Autodesk Inventor part; units mm, degrees
ref_plane "YZ Plane" through (0, 0, 0) normal (1, 0, 0) x (0, 1, 0)
ref_plane "XZ Plane" through (0, 0, 0) normal (0, 1, 0) x (-1, 0, 0)
ref_plane "XY Plane" through (0, 0, 0) normal (0, 0, 1) x (1, 0, 0)
sketch "스케치1" plane through (0, 0, 0) normal (0, 1, 0) x (-1, 0, 0)
  line L0 (0, 0) -> (12, 0)
  line L1 (12, 0) -> (12, -4)
  line L2 (12, -4) -> (0, -4)
  line L3 (0, -4) -> (0, 0)
  dimension "d0" = 12
  dimension "d1" = 4
extrude "돌출1" add sketch "스케치1" along normal blind 3.5
sketch "스케치2" plane through (0, 3.5, 0) normal (0, 1, 0) x (1, 0, 0)
  line L0 (0, 0) -> (0, 4) construction
  line L1 (0, 2) -> (-12, 2) construction
  line L2 (-12, 4) -> (-12, 0) construction
  point P0 (-1.3, 2)
  point P1 (-7.7, 2)
  point P2 (-10.7, 2)
  dimension "d59" = 1.3
  dimension "d60" = 3
  dimension "d62" = 1.3
hole "구멍1" at (-10.7, 3.5, -2) at (-1.3, 3.5, -2) direction (0, -1, 0) diameter 1.1 end through all
hole "구멍2" at (-7.7, 3.5, -2) direction (0, -1, 0) diameter 1.1 end through all
sketch "스케치11" plane through (0, 0, -4) normal (0, 0, -1) x (-1, 0, 0)
  line L0 (0, 0) -> (12, 0)
  line L1 (0, 0) -> (0, 3.5)
  line L2 (12, 3.5) -> (0, 3.5)
  line L3 (12, 0) -> (12, 3.5)
  line L4 (12, 3.5) -> (0, 3.5)
  line L5 (2.5, 3.5) -> (4.1, 3.5)
  line L6 (4.1, 3.5) -> (4.1, -4)
  line L7 (4.1, -4) -> (2.5, -4)
  line L8 (2.5, -4) -> (2.5, 3.5)
  dimension "d99" = 1.6
  dimension "d100" = 4
  dimension "d124" = 2.5
extrude "돌출9" add sketch "스케치11" along normal blind 1.5 contours L8 L2 L6 L0 | L0 L6 L7 L8
chamfer "모따기6" distance 1 angle 45 2 edges at (-2.5, 1.75, -4) (-4.1, 1.75, -4)
chamfer "모따기7" distance 0.5 angle 45 2 edges at (-2.5, 0, -4.5) (-4.1, 0, -4.5)
sketch "스케치12" plane through (0, 0, -5.5) normal (0, 0, -1) x (-1, 0, 0)
  line L0 (4.1, 3.5) -> (2.5, 3.5)
  line L1 (2.5, 3.5) -> (2.5, -4)
  line L2 (2.5, -4) -> (4.1, -4)
  line L3 (4.1, -4) -> (4.1, 3.5)
  line L4 (2.8, -4) -> (2.8, 3.5)
  line L5 (12, 3.5) -> (0, 3.5)
  line L6 (3.8, 3.5) -> (3.8, -4)
  line L7 (2.5, -4) -> (4.1, -4)
  point P0 (0, 0)
  point P1 (3.8, -4)
  dimension "d110" = 1
  dimension "d111" = 0.3
  dimension "d112" = 0.3
extrude "돌출10" cut sketch "스케치12" against normal blind 0.2 contours L6 L2 L4 L0
sketch "스케치13" plane through (0, 0, -4) normal (0, 0, 1) x (1, 0, 0)
  line L0 (-4.6, 0) -> (-2, 0)
  line L1 (-4.1, -0.5) -> (-4.6, 0)
  line L2 (-4.1, -4) -> (-4.1, -0.5)
  line L3 (-2.5, -4) -> (-4.1, -4)
  line L4 (-2.5, -0.5) -> (-2.5, -4)
  line L5 (-2, 0) -> (-2.5, -0.5)
  point P0 (0, 0)
extrude "돌출11" cut sketch "스케치13" against normal blind 0.5
chamfer "모따기8" distance 0.5 distance2 1 1 edges at (-3.3, -4, -4.5) measured on face at (-3.1333, -4, -4.7667)
sketch "스케치14" plane through (-12, 0, 0) normal (0, 0, 1) x (1, 0, 0)
  line L0 (12, 0) -> (0, 0)
  line L1 (12, 0) -> (12, 3.5)
  line L2 (0, 3.5) -> (12, 3.5)
  line L3 (0, 0) -> (0, 3.5)
extrude "돌출12" cut sketch "스케치14" against normal blind 0.5
equation "\"d111\" = d112"
equation "\"G23_F\" = 0.65"
equation "\"G23_M\" = 0.67"
equation "\"Screw_F\" = 1.3"
equation "\"Screw_M\" = 1.6"
properties part number "_3D 인쇄"
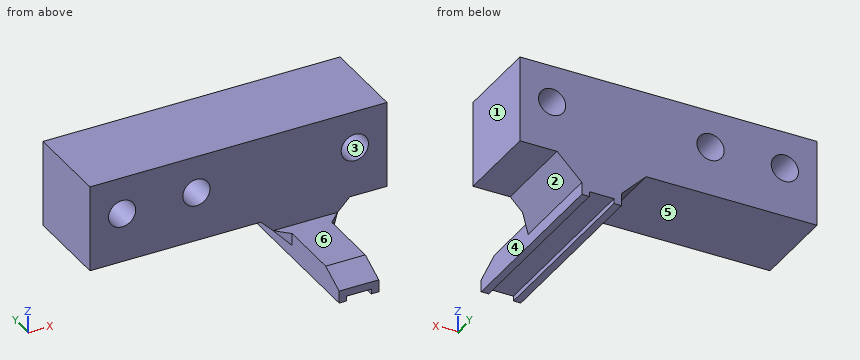
Verification items for the finished model (mm, model axes). Face numbers are marked on the shaded views. A direction names the side the tool comes from. Coordinates: 2 decimals unless noted, no trailing zeros. Order: outer loops, then holes, each group sorted by start corner. A loop starts at its lowest first (then second) coordinate and runs counter-clockwise, first axis right, second up. Notation, with made-up numbers: M 72.25,-35 L 130.25,-35 A37 cw 130.25,4 Z; hole C 60.25,-17 d2. An arc over 180 degrees is marked long. One line per item, written item: value. Start each with the question number.
Item 1: Sectioned sample at A-A (z = -2). Enter the section's corners in (x, y).
Item 2: Sectioned sample at C-C (y = -1). Enter the section's corners in (x, z).
Item 3: Scan lines: probe 1 along X at (y, z) = (2.65, -2); probe 2 along Z at (x, y) = (-10.7, 1.05); probe 3 along Z at (x, y) = (-7, 2). Record each from-to range of solid material in increasing order.
Item 4: Mould release check, pull along Z, two halves, no side actions. Record for the marked faces 1, 2 and 3: released by +Z, released by -Z, zero draft, split by the parting line, or undercut.
Item 5: Sectioned sample at B-B (x = -10.7). Enter the section's corners in (y, z), then the cut area to 3 significant figures.
Item 6: Gauge pin test, flat ends, axial feed: pin 1 (1.8 mm diameter, centred on x = -8, y = 2, fed in from -Z); pin 2 (3 mm diameter, centred on x = -3.5, y = -2, fed in from +Z); pin 3 (0.5 mm diameter, centred on y = -1.5, z = -5, fed in from -X). Record the tip position at first contact, or that the pin passes through.
Item 7: Access from +Z, -Z, +X, -X, +Y, -Y to the whole of each face (thin tool, end or side, straight path). Record for the marked faces 4, 5 and 6.
Item 8: Sectioned sample at D-D (y = 2.5). Enter the section's corners in (x, z), then the cut area to 3 significant figures.
Conclusion:
1. outline: M -12,0 L -11.25,0 L -11.25,3.5 L -12,3.5 Z; M -10.15,0 L -8.25,0 L -8.25,3.5 L -10.15,3.5 Z; M -7.15,0 L -1.85,0 L -1.85,3.5 L -7.15,3.5 Z; M -0.75,0 L 0,0 L 0,3.5 L -0.75,3.5 Z
2. outline: M -4.1,-5.5 L -3.8,-5.5 L -3.8,-5.3 L -2.8,-5.3 L -2.8,-5.5 L -2.5,-5.5 L -2.5,-4.5 L -4.1,-4.5 Z
3. probe 1: x = -12 to -11.25, -10.15 to -8.25, -7.15 to -1.85, -0.75 to 0
3. probe 2: z = -4 to -2.55, -1.45 to -0.5
3. probe 3: z = -4 to -0.5
4. face 1: zero draft
4. face 2: released by -Z
4. face 3: undercut
5. outline: M 0,-4 L 3.5,-4 L 3.5,-2.55 L 0,-2.55 Z; M 0,-1.45 L 3.5,-1.45 L 3.5,-0.5 L 0,-0.5 Z
5. area: 8.40 mm^2
6. pin 1: stops at z = -4
6. pin 2: stops at z = -4.5
6. pin 3: stops at x = -4.1
7. face 4: -Z, +X, -Y
7. face 5: -Z, -X, +Y, -Y
7. face 6: +Z, +X, -X, -Y
8. outline: M -12,-4 L -5.1,-4 L -4.1,-5 L -4.1,-5.5 L -3.8,-5.5 L -3.8,-5.3 L -2.8,-5.3 L -2.8,-5.5 L -2.5,-5.5 L -2.5,-5 L -1.5,-4 L 0,-4 L 0,-0.5 L -12,-0.5 Z; hole C -10.7,-2 d1.1; hole C -7.7,-2 d1.1; hole C -1.3,-2 d1.1
8. area: 42.3 mm^2
